from build123d import *

# Parameters (mm, degrees)
SKETCH100_W             = 50
SKETCH100_H             = 50
PAD017_DEPTH            = 20
POCKET084_DEPTH         = 20.001
POCKET085_DEPTH         = 50.001
POCKET086_DEPTH         = 50.001
SKETCH104_R             = 1.55
POCKET087_DEPTH         = 5
SKETCH105_R             = 1.55
POCKET088_DEPTH         = 3
SKETCH106_R             = 1.55
POCKET089_DEPTH         = 3
BODY018_PLACEMENT_ANGLE = 90


with BuildPart() as part:
    # Sketch100 → Pad017 (new body)
    with BuildSketch(Plane.XY):
        Rectangle(SKETCH100_W, SKETCH100_H)
    extrude(amount=PAD017_DEPTH)

    # Sketch101 (on Face6 of Pad017) → Pocket084 (cut, through all)
    with BuildSketch(Plane.XY.offset(20)):
        with BuildLine():
            Line((-18, 15), (-17, 15))
            ThreePointArc((-17, 15), (-15.585786, 15.585786), (-15, 17))
            Line((-15, 17), (-15, 18))
            ThreePointArc((-13, 20), (-14.414214, 19.414214), (-15, 18))
            Line((-13, 20), (13, 20))
            ThreePointArc((15, 18), (14.414214, 19.414214), (13, 20))
            Line((15, 18), (15, 17))
            ThreePointArc((15, 17), (15.585786, 15.585786), (17, 15))
            Line((17, 15), (18, 15))
            ThreePointArc((20, 13), (19.414214, 14.414214), (18, 15))
            Line((20, 13), (20, -13))
            ThreePointArc((18, -15), (19.414214, -14.414214), (20, -13))
            Line((18, -15), (17, -15))
            ThreePointArc((17, -15), (15.585786, -15.585786), (15, -17))
            Line((15, -17), (15, -18))
            ThreePointArc((13, -20), (14.414214, -19.414214), (15, -18))
            Line((13, -20), (-13, -20))
            ThreePointArc((-15, -18), (-14.414214, -19.414214), (-13, -20))
            Line((-15, -18), (-15, -17))
            ThreePointArc((-15, -17), (-15.585786, -15.585786), (-17, -15))
            Line((-17, -15), (-18, -15))
            ThreePointArc((-20, -13), (-19.414214, -14.414214), (-18, -15))
            Line((-20, -13), (-20, 13))
            ThreePointArc((-18, 15), (-19.414214, 14.414214), (-20, 13))
        make_face()
    extrude(amount=-POCKET084_DEPTH, mode=Mode.SUBTRACT)

    # Sketch102 (on Face3 of Pocket084) → Pocket085 (cut, through all)
    with BuildSketch(Plane.YZ.offset(25)):
        with BuildLine():
            Line((-15, 10), (15, 10))
            ThreePointArc((20, 5), (18.535534, 8.535534), (15, 10))
            Line((20, 5), (20, 0))
            Line((20, 0), (-20, 0))
            Line((-20, 0), (-20, 5))
            ThreePointArc((-15, 10), (-18.535534, 8.535534), (-20, 5))
        make_face()
    extrude(amount=-POCKET085_DEPTH, mode=Mode.SUBTRACT)

    # Sketch103 (on Face6 of Pocket084) → Pocket086 (cut, through all)
    with BuildSketch(Plane.XZ.offset(25)):
        with BuildLine():
            Line((-15, 10), (15, 10))
            ThreePointArc((20, 5), (18.535534, 8.535534), (15, 10))
            Line((20, 5), (20, 0))
            Line((20, 0), (-20, 0))
            Line((-20, 0), (-20, 5))
            ThreePointArc((-15, 10), (-18.535534, 8.535534), (-20, 5))
        make_face()
    extrude(amount=-POCKET086_DEPTH, mode=Mode.SUBTRACT)

    # Sketch104 → Pocket087 (cut)
    with BuildSketch(Plane.XY.offset(20)):
        with Locations((-20, 20)):
            Circle(SKETCH104_R)
        with Locations((20, 20)):
            Circle(SKETCH104_R)
        with Locations((20, -20)):
            Circle(SKETCH104_R)
        with Locations((-20, -20)):
            Circle(SKETCH104_R)
    extrude(amount=-POCKET087_DEPTH, mode=Mode.SUBTRACT)

    # Sketch105 (on Face27 of Pocket087) → Pocket088 (cut)
    with BuildSketch(Plane.XZ.offset(25)):
        with Locations((-20, 14)):
            Circle(SKETCH105_R)
        with Locations((20, 14)):
            Circle(SKETCH105_R)
    extrude(amount=-POCKET088_DEPTH, mode=Mode.SUBTRACT)

    # Sketch106 (on Face11 of Pocket088) → Pocket089 (cut)
    with BuildSketch(Plane(origin=(-25, 0, 0), x_dir=(0, -1, 0), z_dir=(-1, 0, 0))):
        with Locations((-20, 14)):
            Circle(SKETCH106_R)
        with Locations((20, 14)):
            Circle(SKETCH106_R)
    extrude(amount=-POCKET089_DEPTH, mode=Mode.SUBTRACT)


with BuildPart() as part_1:
    # Body018 placement: moved
    add(part.part.moved(Location((145, 25, 0))).rotate(Axis((145, 25, 0), (0, 0, 1)), BODY018_PLACEMENT_ANGLE))


solid = part_1.part
Design review of the part built by this model. Coordinates are the model's own, in mm. A direction names the side the tool comes from. Give positions to 0.01 mm unless a question says otherwise; leave off trailing zeros. Order: outer loops, then holes, each group sorted by start corner. A loop starts at its lowest first (then second) coordinate and runs counter-clockwise, first axis right, second up. Notation, with made-up numbers: (57, 34.25) - (73, 34.25) arc R34 cw to (73, 70.25) - close; hole circle Ø2 at (-20.75, 69.5). An arc over 180 degrees is marked (long way). Use CSV: the item, a comma, the result in double quotes. Start each with the question number.
Q1. For P1, Ø0.9, axis at x = 164.5, y = 4.5, coming from the +Z side; P2, Ø2, axis at x = 123, y = 19.5, coming from the -Z side, all flat-tipped, find the tip position at first contact; note any pin that passes through.
Q2. Take a section at C-C (y = 30). State the section outline as (x, z) points.
Q3. For line 1 (Y direction, x = 152, z = 12.75); line 2 (X direction, y = 32, z = 16.5); line 3 (Y direction, x = 166, z = 18), list the stretches that pass through material, from the lowest coordinate up.
Q4. Take a section at D-D (z = 7.5). State the section outline as (x, y) points, and give its area (3 significant figures).
Q5. Machinability: for faces 4 (the face through (123.45, 1.48, 14.07)), 5 (the face through (165, 5, 15)), 6 (the face through (159.4, 5.57, 15.07)), 7 (the face through (124, 7, 9)), 8 (the face through (127, 46, 9)), which of the approach directions +Z, -Z, +X, -X, +Y, -Y give a long, thin tool a straight path to every point of the face, cutting with its end or side? Answer none if there is none.
Q6. Take a section at A-A (z = 17). Count the separate pieces of the cut face and the enclosed holes in it, and give its area (3 significant figures).
Q7. Take a section at B-B (x = 140.5). State the section outline as (y, z) points.
Q8. Draft analysis for pull direction Y (two halves, no side actions). For faces 1 (the face through (145, 0, 12)), 2 (the face through (166, 7, 9)), 3 (the face through (170, 25, 12)), state which applies: pulls with the +Y half, pulls with the -Y half, needs draft (parallel to the pull), parting line crosses it, or undercut.
Calculated:
1,P1,"stops at z = 15"
1,P2,"stops at z = 10"
2,outline,"(120, 10) - (125, 10) - (125, 20) - (120, 20) - close; (165, 10) - (170, 10) - (170, 20) - (165, 20) - close"
3,line 1,"y = 0 to 5, 45 to 50"
3,line 2,"x = 120 to 125, 165 to 170"
3,line 3,"y = 0 to 3.82, 6.18 to 43.82, 46.18 to 50"
4,outline,"(120, 0) - (125.67, 0) - (125.67, 5.67) - (120, 5.67) - close; (120, 44.33) - (125.67, 44.33) - (125.67, 50) - (120, 50) - close; (164.33, 0) - (170, 0) - (170, 5.67) - (164.33, 5.67) - close; (164.33, 44.33) - (170, 44.33) - (170, 50) - (164.33, 50) - close"
4,area,"129 mm²"
5,face 4,"-Y"
5,face 5,"+Z"
5,face 6,"+Z, -Z"
5,face 7,"-Z, +X, -X"
5,face 8,"-Z, +Y, -Y"
6,separate pieces,"1"
6,enclosed holes,"5"
6,area,"973 mm²"
7,outline,"(0, 10) - (5, 10) - (5, 20) - (0, 20) - close; (45, 10) - (50, 10) - (50, 20) - (45, 20) - close"
8,face 1,"pulls with the -Y half"
8,face 2,"undercut"
8,face 3,"needs draft"
